Here's how the part is built. I have some questions about the finished solid (model axes, mm). Round coordinates to 2 decimals unless told otherwise and drop trailing zeros. Order: outer loops, then holes, each group sorted by start corner. A loop starts at its lowest first (then second) coordinate and runs counter-clockwise, first axis right, second up. Notation, with made-up numbers: (-28, 83.5) - (-12, 83.5) arc R22 ccw to (-12, 97.5) - close; hole circle Ø9 at (46, 26). An arc over 180 degrees is marked (long way). One line per item, written item: value.
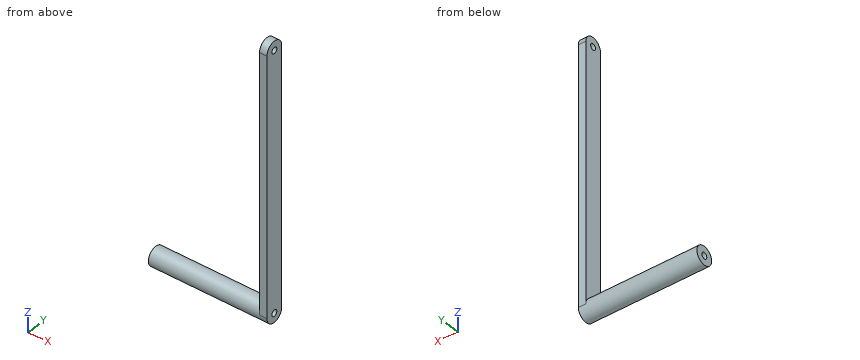
from build123d import *

# Parameters (mm, degrees)
RESSALTO_EXTRUS_O1_DEPTH = 2
RESSALTO_EXTRUS_O2_START = 30
ESBO_O2_R                = 2.5
RESSALTO_EXTRUS_O2_DEPTH = 30
CORTE_EXTRUS_O1_REACH    = 51.361
ESBO_O3_R                = 0.85
CORTE_EXTRUS_O2_REACH    = 50.088
ESBO_O4_R                = 0.85


with BuildPart() as part:
    # Esboço1 → Ressalto-extrusão1 (new body)
    with BuildSketch(Plane(origin=(0, 0, 0), x_dir=(0, 0, -1), z_dir=(1, 0, 0))):
        with BuildLine():
            Line((-35, 2.5), (35, 2.5))
            ThreePointArc((35, 2.5), (37.5, 0), (35, -2.5))
            Line((35, -2.5), (-35, -2.5))
            ThreePointArc((-35, -2.5), (-37.5, 0), (-35, 2.5))
        make_face()
    extrude(amount=RESSALTO_EXTRUS_O1_DEPTH)

    # Esboço2 → Ressalto-extrusão2 (add)
    with BuildSketch(Plane.ZY.offset(RESSALTO_EXTRUS_O2_START)):
        with Locations((-35, 0)):
            Circle(ESBO_O2_R)
    extrude(amount=-RESSALTO_EXTRUS_O2_DEPTH)

    # Esboço3 → Corte-extrusão1 (cut, up to next)
    with BuildSketch(Plane.ZY.offset(30), mode=Mode.PRIVATE) as corte_extrus_o1_sk1:
        with Locations((-35, 0)):
            Circle(ESBO_O3_R)
    corte_extrus_o1_tool1 = extrude(corte_extrus_o1_sk1.sketch, amount=-CORTE_EXTRUS_O1_REACH, mode=Mode.PRIVATE) & part.part
    add(corte_extrus_o1_tool1.solids().sort_by_distance((-30, 0, -35))[0], mode=Mode.SUBTRACT)

    # Esboço4 → Corte-extrusão2 (cut, up to next)
    with BuildSketch(Plane.ZY, mode=Mode.PRIVATE) as corte_extrus_o2_sk1:
        with Locations((35, 0)):
            Circle(ESBO_O4_R)
    corte_extrus_o2_tool1 = extrude(corte_extrus_o2_sk1.sketch, amount=-CORTE_EXTRUS_O2_REACH, mode=Mode.PRIVATE) & part.part
    add(corte_extrus_o2_tool1.solids().sort_by_distance((0, 0, 35))[0], mode=Mode.SUBTRACT)


solid = part.part
Q1. If we section it at B-B, the plane x = -3: Please give me the cut outline in (y, z).
Results list:
outline: circle Ø5 at (0, -35); hole circle Ø1.7 at (0, -35)
Q2. If I drill on line 1 along Z through (x, y) = (-9.5, 0.05); line 2 along Y through (x, z) = (1.55, 35); line 3 along X through (y, z) = (0.95, 34.5), over which ranges is the centre line in solid material (lowest first)?
Results list:
line 1: -37.5 to -35.85, -34.15 to -32.5
line 2: -2.5 to -0.85, 0.85 to 2.5
line 3: 0 to 2
Q3. Will these pins go through, and if not, where does the flat tip stop? pin 1 (5 mm diameter, centred on x = -3, z = -6.5, fed in from +Y); pin 2 (1.5 mm diameter, centred on y = -1, z = 13.5, fed in from -X); pin 3 (3 mm diameter, centred on x = -2, y = -2, fed in from +Z); pin 4 (2.5 mm diameter, centred on y = 0, z = -35, fed in from +X).
Results list:
pin 1: through
pin 2: x = 0
pin 3: z = -32.55
pin 4: x = 2
Q4. If we section it at C-C, the plane z = 20.5: Please give me the cut outline in (x, y), then the cut area to 3 significant figures.
Results list:
outline: (0, -2.5) - (2, -2.5) - (2, 2.5) - (0, 2.5) - close
area: 10.0 mm²
Q5. If we section it at A-A, the plane y = 0: Please give me the cut outline in (x, z), then the cut area to 3 significant figures.
Results list:
outline: (-30, -37.5) - (2, -37.5) - (2, -35.85) - (-30, -35.85) - close; (-30, -34.15) - (2, -34.15) - (2, 34.15) - (0, 34.15) - (0, -32.5) - (-30, -32.5) - close; (0, 35.85) - (2, 35.85) - (2, 37.5) - (0, 37.5) - close
area: 242 mm²
